Verification items for this drawing (mm, ordinates from the low corner). Round coordinates to 2 decimals unless told otherwise and drop trailing zeros. Order: outer loops, then holes, each group sorted by start corner. A loop starts at its lowest first (then second) coordinate and runs counter-clockwise, first axis right, second up. Notation, with made-up numbers: M 61.25,-38.5 L 113.25,-38.5 A22 cw 113.25,-4.5 Z; hole C -39.75,8.5 d2. An arc over 180 degrees is marked long. Use CSV: the item, a comma, the result in double quotes. Start each with the question number.
Q1. Scan lines: line 1 (X direction, y = 2.25, z = 114.5); line 2 (Z direction, x = 62, y = 2); line 3 (Y direction, x = 35, z = 64). Record each from-to range of solid material in increasing order.
Q2. Sectioned sample at C-C (z = 125.5). Enter the section's corners in (x, y) (1 decimal), and give its area (3 significant figures).
Q3. Sectioned sample at A-A (x = 19.5). Enter the section's corners in (y, z).
Q4. Gauge pin test, flat end, axial feed: pin 1 Ø6 at (x, z) = (7.5, 91) entering from -Y. Record the tip position at first contact, or that the pin passes through.
Q5. Mould release check, pull along Z, two halves, no side actions. Record for the marked faces 1 and 2: +Z half, -Z half, draft (parallel to the pull), parting line (faces both ways), or undercut.
Q6. Sectioned sample at D-D (z = 97). Enter the section's corners in (x, y), and give its area (3 significant figures).
Q7. Sectioned sample at B-B (y = 2.5). Enter the section's corners in (x, z).
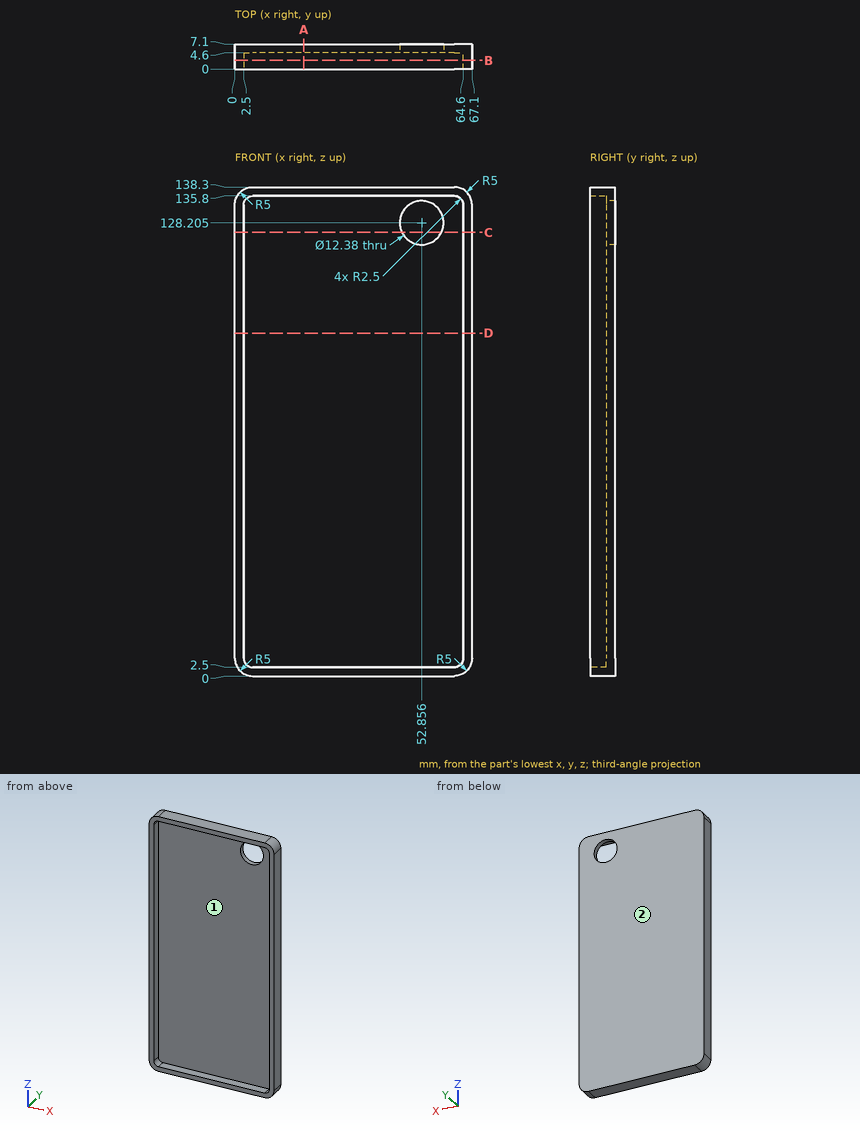
Verdict:
1,line 1,"x = 0 to 2.5, 64.6 to 67.1"
1,line 2,"z = 0 to 2.5, 135.8 to 138.3"
1,line 3,"y = 4.6 to 7.1"
2,outline,"M 0,0 L 2.5,0 L 2.5,4.6 L 47.3,4.6 L 47.3,7.1 L 0,7.1 Z; M 58.4,4.6 L 64.6,4.6 L 64.6,0 L 67.1,0 L 67.1,7.1 L 58.4,7.1 Z"
2,area,"163 mm²"
3,outline,"M 0,0 L 7.1,0 L 7.1,138.3 L 0,138.3 L 0,135.8 L 4.6,135.8 L 4.6,2.5 L 0,2.5 Z"
4,pin 1,"stops at y = 4.6"
5,face 1,"undercut"
5,face 2,"draft"
6,outline,"M 0,0 L 2.5,0 L 2.5,4.6 L 64.6,4.6 L 64.6,0 L 67.1,0 L 67.1,7.1 L 0,7.1 Z"
6,area,"191 mm²"
7,outline,"M 0,5 A5 ccw 5,0 L 62.1,0 A5 ccw 67.1,5 L 67.1,133.3 A5 ccw 62.1,138.3 L 5,138.3 A5 ccw 0,133.3 Z; hole M 2.5,5 A2.5 ccw 5,2.5 L 62.1,2.5 A2.5 ccw 64.6,5 L 64.6,133.3 A2.5 ccw 62.1,135.8 L 5,135.8 A2.5 ccw 2.5,133.3 Z"
